```python
from build123d import *

# Parameters (mm, degrees)
SKETCH1_R           = 0.440528634
BOSS_EXTRUDE1_DEPTH = 1.2


with BuildPart() as part:
    # Sketch1 → Boss-Extrude1 (new body)
    with BuildSketch(Plane(origin=(0.6, 0, 0), x_dir=(0, 0, -1), z_dir=(1, 0, 0))):
        with BuildLine():
            Line((-1.406616674, -4.833075449), (-1.361950738, -4.679605182))
            ThreePointArc((-1.361950738, -4.679605182), (-1.693445711, -3.612076228), (-2.805550353, -3.499247827))
            ThreePointArc((-2.805550353, -3.499247827), (-3.517808728, -3.586040603), (-4.108949504, -3.179349612))
            ThreePointArc((-4.108949504, -3.179349612), (0, 4.669603524), (4.108949504, -3.179349612))
            ThreePointArc((4.108949504, -3.179349612), (3.517808728, -3.586040603), (2.805550353, -3.499247827))
            ThreePointArc((2.805550353, -3.499247827), (1.693445711, -3.612076228), (1.361950738, -4.679605182))
            Line((1.361950738, -4.679605182), (1.406616674, -4.833075449))
            ThreePointArc((1.406616674, -4.833075449), (1.89690358, -5.392945454), (2.640948929, -5.377707645))
            ThreePointArc((2.640948929, -5.377707645), (0, 5.991189427), (-2.640948929, -5.377707645))
            ThreePointArc((-2.640948929, -5.377707645), (-1.89690358, -5.392945454), (-1.406616674, -4.833075449))
        make_face()
        with Locations((-2.334801762, -4.396466943)):
            Circle(SKETCH1_R, mode=Mode.SUBTRACT)
        with Locations((2.334801762, -4.396466943)):
            Circle(SKETCH1_R, mode=Mode.SUBTRACT)
    extrude(amount=-BOSS_EXTRUDE1_DEPTH)


solid = part.part
```
Design review of the part built by this model. Coordinates are the model's own, in mm. Give positions to 0.01 mm unless a question says otherwise; leave off trailing zeros. Write each loop counter-clockwise with the first axis right and the second up, starting at its lowest first coordinate (ties: lowest second). Pieces come first, ordered by that corner, then holes.
(1) Clearance check with flat-ended pins moving along their axes: pin 1 Ø4 at (y, z) = (1.5, 2.5) entering from -X; pin 2 Ø4 at (y, z) = (1, 0) entering from +X. State where each tip first meets the part, or that it passes through.
Checked values:
pin 1: stops at x = -0.6
pin 2: passes through
(2) Wall thickness on line 1 along Y through (x, z) = (-0.45, -2.5); line 2 along Y through (x, z) = (-0.05, 2); line 3 along Z through (x, y) = (-0.25, -4.5): over which ranges is each line inside the solid? List them lowest first.
Checked values:
line 1: y = -5.43 to -4.8, -3.99 to -3.4, 4 to 5.44
line 2: y = -5.43 to -4.68, -4.11 to -3.44, 4.25 to 5.65
line 3: z = -3.96 to -2.76, -1.91 to -1.33, 1.33 to 1.91, 2.76 to 3.96
(3) Add section B-B (z = -3.25). Give the boundary of the cut face in (x, y), and give its area (3 significant figures).
Checked values:
outline: (-0.6, -5.03) - (0.6, -5.03) - (0.6, -3.61) - (-0.6, -3.61) - close; (-0.6, 3.47) - (0.6, 3.47) - (0.6, 5.03) - (-0.6, 5.03) - close
area: 3.58 mm2
(4) Add section C-C (x = -0.3). Give the boundary of the cut face in (y, z), and give its area (3 significant figures).
Checked values:
outline: (-5.38, -2.64) arc R5.99 ccw (long way) to (-5.38, 2.64) arc R0.88 ccw to (-4.83, 1.41) - (-4.68, 1.36) arc R1.01 ccw to (-3.5, 2.81) arc R1.01 cw to (-3.18, 4.11) arc R5 cw (long way) to (-3.18, -4.11) arc R1.01 cw to (-3.5, -2.81) arc R1.01 ccw to (-4.68, -1.36) - (-4.83, -1.41) arc R0.88 ccw to start; hole circle Ø0.88 at (-4.4, -2.33); hole circle Ø0.88 at (-4.4, 2.33)
area: 35.3 mm2
(5) Mouldability with a two-part tool opening along Z and no side actions: class faces 1 (the face through (-0.6, 3, 4)), 2 (the face through (0.008, -4.264, -2.755)), 3 (the face through (0.01, -5.4, 1.91)), 4 (the face through (0.008, 5.987, -0.225)) as +Z half, -Z half, draft (parallel to the pull), parting line (faces both ways), or undercut.
Checked values:
face 1: draft
face 2: undercut
face 3: undercut
face 4: parting line
(6) Add section D-D (z = 0). Give the boundary of the cut face in (x, y).
Checked values:
outline: (-0.6, 4.67) - (0.6, 4.67) - (0.6, 5.99) - (-0.6, 5.99) - close
(7) Add section A-A (y = -0.25). Give the boundary of the cut face in (x, z), and give its area (3 significant figures).
Checked values:
outline: (-0.6, -5.99) - (0.6, -5.99) - (0.6, -5) - (-0.6, -5) - close; (-0.6, 5) - (0.6, 5) - (0.6, 5.99) - (-0.6, 5.99) - close
area: 2.37 mm2
